The model under review builds one solid part; all positions refer to its coordinate system, in mm. Coordinates: 2 decimals unless noted, no trailing zeros. Loops run counter-clockwise (first coordinate to the right, second up) from the corner with the lowest first, then second, coordinate; pieces in that order, holes last. Notation, with made-up numbers: M 54,44 L 105,44 A14 cw 105,55 Z; hole C 83,81 d2. An arc over 180 degrees is marked long. Use one line per item in the form item = value.
```python
from build123d import *

# Parameters (mm, degrees)
SKETCH1_W           = 18.796
SKETCH1_H           = 18.796
BOSS_EXTRUDE1_DEPTH = 63.5
FILLET1_R           = 3.175
SKETCH2_R           = 2.5527
CUT_EXTRUDE1_DEPTH  = 63.5
SKETCH3_R           = 2.5527
CUT_EXTRUDE2_DEPTH  = 63.5


with BuildPart() as part:
    # Sketch1 → Boss-Extrude1 (new body)
    with BuildSketch(Plane.XY):
        with Locations((9.398, 9.398)):
            Rectangle(SKETCH1_W, SKETCH1_H)
    extrude(amount=BOSS_EXTRUDE1_DEPTH)

    # Fillet1
    fillet1_edges = [part.edges().sort_by_distance(p)[0] for p in [
        (0, 18.796, 31.75),
        (18.796, 18.796, 31.75),
        (18.796, 0, 31.75),
        (0, 0, 31.75),
    ]]
    fillet(fillet1_edges, radius=FILLET1_R)

    # Sketch2 → Cut-Extrude1 (cut)
    with BuildSketch(Plane(origin=(0, 18.796, 0), x_dir=(1, 0, 0), z_dir=(0, 1, 0))):
        with Locations(Location((9.398, -6.35, 0), (0, 0, 270))):
            Circle(SKETCH2_R)
        with Locations(Location((9.398, -19.05, 0), (0, 0, 270))):
            Circle(SKETCH2_R)
        with Locations(Location((9.398, -31.75, 0), (0, 0, 270))):
            Circle(SKETCH2_R)
        with Locations(Location((9.398, -44.45, 0), (0, 0, 270))):
            Circle(SKETCH2_R)
        with Locations(Location((9.398, -57.15, 0), (0, 0, 270))):
            Circle(SKETCH2_R)
    extrude(amount=-CUT_EXTRUDE1_DEPTH, mode=Mode.SUBTRACT)

    # Sketch3 → Cut-Extrude2 (cut)
    with BuildSketch(Plane(origin=(18.796, 0, 0), x_dir=(0, 0, -1), z_dir=(1, 0, 0))):
        with Locations(Location((-57.15, 9.398, 0), (0, 0, 90))):
            Circle(SKETCH3_R)
        with Locations(Location((-44.45, 9.398, 0), (0, 0, 90))):
            Circle(SKETCH3_R)
        with Locations(Location((-31.75, 9.398, 0), (0, 0, 90))):
            Circle(SKETCH3_R)
        with Locations(Location((-19.05, 9.398, 0), (0, 0, 90))):
            Circle(SKETCH3_R)
        with Locations(Location((-6.35, 9.398, 0), (0, 0, 90))):
            Circle(SKETCH3_R)
    extrude(amount=-CUT_EXTRUDE2_DEPTH, mode=Mode.SUBTRACT)


solid = part.part
```
1. Add section D-D (z = 26). State the section outline as (x, y) points (3 decimals), then the cut area to 3 significant figures.
Response values:
outline = M 0,3.175 A3.175 ccw 3.175,0 L 15.621,0 A3.175 ccw 18.796,3.175 L 18.796,15.621 A3.175 ccw 15.621,18.796 L 3.175,18.796 A3.175 ccw 0,15.621 Z
area = 345 mm^2
2. Add section B-B (y = 5.5). State the section outline as (x, z) points, then the cut area to 3 significant figures.
Response values:
outline = M 0,0 L 18.8,0 L 18.8,63.5 L 0,63.5 Z; hole C 9.4,6.35 d5.11; hole C 9.4,19.05 d5.11; hole C 9.4,31.75 d5.11; hole C 9.4,44.45 d5.11; hole C 9.4,57.15 d5.11
area = 1,090 mm^2
3. The part is to be moulded in two halves that separate along X. For faces 1 (the face through (18.796, 6.5, 31.3)), 2 (the face through (0, 6.5, 31.3)), 3 (the face through (6.5, 18.796, 31.3)), 4 (the face through (9.5, 3.7, 54.6)), say which applies: pulls with the +X half, pulls with the -X half, needs draft (parallel to the pull), parting line crosses it, or undercut.
Response values:
face_1 = pulls with the +X half
face_2 = pulls with the -X half
face_3 = needs draft
face_4 = undercut
4. Wall thickness on line 1 along Z through (x, y) = (5.75, 9.5); line 2 along Y through (x, z) = (3, 19); line 3 along Z through (x, y) = (12.5, 7.25): over which ranges is each line inside the solid? List them lowest first. Write a range as from..to.
Response values:
line_1 = 0..3.8, 8.9..16.5, 21.6..29.2, 34.3..41.9, 47..54.6, 59.7..63.5
line_2 = 0..6.85, 11.95..18.79
line_3 = 0..4.97, 7.73..17.67, 20.43..30.37, 33.13..43.07, 45.83..55.77, 58.53..63.5
5. Add section A-A (z = 19.05). State the section outline as (x, y) points (3 decimals), then the cut area to 3 significant figures.
Response values:
outline = M 0,3.175 A3.175 ccw 3.175,0 L 6.845,0 L 6.845,6.845 L 0,6.845 Z; M 0,11.951 L 6.845,11.951 L 6.845,18.796 L 3.175,18.796 A3.175 ccw 0,15.621 Z; M 11.951,0 L 15.621,0 A3.175 ccw 18.796,3.175 L 18.796,6.845 L 11.951,6.845 Z; M 11.951,11.951 L 18.796,11.951 L 18.796,15.621 A3.175 ccw 15.621,18.796 L 11.951,18.796 Z
area = 179 mm^2
